For this review, take the finished solid that the model builds, in its own axes (mm). Round coordinates to 2 decimals unless told otherwise and drop trailing zeros. Write each loop counter-clockwise with the first axis right and the second up, starting at its lowest first coordinate (ties: lowest second). Pieces come first, ordered by that corner, then holes. Notation, with made-up numbers: M 18,8.5 L 53,8.5 A30 ccw 53,46.5 Z; hole C -37.5,50 d5. An arc over 180 degrees is marked long. Write each question's results on one line, items separated by ' | '. Start each with the question number.
```python
from build123d import *

# Parameters (mm, degrees)
BOSS_EXTRUDE1_DEPTH       = 1.5
FILLET1_R                 = 4
F_3_0MM_DOWEL_HOLE2_D     = 3
F_3_0MM_DOWEL_HOLE2_DEPTH = 17.29
F_3_0MM_DOWEL_HOLE2_TIP   = 0.901290929


with BuildPart() as part:
    # Sketch1 → Boss-Extrude1 (new body)
    with BuildSketch(Plane(origin=(0, 0, 0), x_dir=(0, 0, -1), z_dir=(1, 0, 0))):
        with BuildLine():
            Line((164.111754286, 40.215722327), (-6.393348286, 40.215722327))
            ThreePointArc((-6.393348286, 40.215722327), (12.614416769, 26.195971709), (19.859203, 3.715722327))
            ThreePointArc((19.859203, 3.715722327), (12.614416769, -18.764527055), (-6.393348286, -32.784277673))
            Line((-6.393348286, -32.784277673), (164.111754286, -32.784277673))
            ThreePointArc((164.111754286, -32.784277673), (137.859203, 3.715722327), (164.111754286, 40.215722327))
        make_face()
    extrude(amount=BOSS_EXTRUDE1_DEPTH)

    # Fillet1
    fillet1_edges = [part.edges().sort_by_distance(p)[0] for p in [
        (0.75, -32.784277673, -164.111754286),
        (0.75, -32.784277673, 6.393348286),
        (0.75, 40.215722327, 6.393348286),
        (0.75, 40.215722327, -164.111754286),
    ]]
    fillet(fillet1_edges, radius=FILLET1_R)

    # Ø3.0mm Dowel Hole2
    with Locations(Plane(origin=(1.5, 0, 0), x_dir=(0, 0, -1), z_dir=(1, 0, 0))):
        with Locations((8.745330875, 36.215722327), (148.973075124, 36.215722327), (148.973075124, -28.784277673), (8.745330875, -28.784277673), (43.745330875, 36.215722327), (113.973075124, -28.784277673)):
            Hole(F_3_0MM_DOWEL_HOLE2_D / 2, depth=F_3_0MM_DOWEL_HOLE2_DEPTH)
            with Locations((0, 0, -(F_3_0MM_DOWEL_HOLE2_DEPTH + F_3_0MM_DOWEL_HOLE2_TIP / 2))):  # 118° drill point
                Cone(0, F_3_0MM_DOWEL_HOLE2_D / 2, F_3_0MM_DOWEL_HOLE2_TIP, mode=Mode.SUBTRACT)


solid = part.part
```
Item 1: We need section C-C on y = 31. State the section outline as (x, z) points.
Item 2: Mouldability with a two-part tool opening along Z and no side actions: class faces 1 (the flat face through (0, 4, -78)), 2 (the cylindrical face through (0.74, -29.36, -112.59)), 3 (the cylindrical face through (0.74, 3.246, -137.862)) as pulls with the +Z half, pulls with the -Z half, needs draft (parallel to the pull), parting line crosses it, or undercut.
Item 3: We need section B-B on y = 0.5. State the section outline as (x, z) points, then the cut area to 3 significant figures.
Item 4: Insertion check: P1, Ø2.5, axis at y = 36.22, z = -43.75, coming from the +X side. The pin has a flat end and moves straight along its axis. Give the tip position at first contact, or say it passes through.
Item 5: We need section A-A on x = 1. State the section outline as (y, z) points.
Item 6: For probe 1 along Y at (x, z) = (1, -16); probe 2 along Y at (x, z) = (0.2, -142.5); probe 3 along Z at (x, y) = (0.7, -14), list the stretches that pass through material, from the lowest coordinate up.
Numbers:
1) outline: M 0,-149.2 L 1.5,-149.2 L 1.5,-8.52 L 0,-8.52 Z
2) face 1: needs draft | face 2: undercut | face 3: pulls with the -Z half
3) outline: M 0,-137.99 L 1.5,-137.99 L 1.5,-19.72 L 0,-19.72 Z | area: 177 mm^2
4) P1: passes through
5) outline: M -32.78,-148.97 A4 ccw -25.73,-151.55 A38.5 cw 33.16,-151.55 A4 ccw 40.22,-148.97 L 40.22,-8.75 A4 ccw 33.16,-6.17 A38.5 cw -25.73,-6.17 A4 ccw -32.78,-8.75 Z; hole C -28.78,-148.97 d3; hole C -28.78,-113.97 d3; hole C -28.78,-8.75 d3; hole C 36.22,-148.97 d3; hole C 36.22,-43.75 d3; hole C 36.22,-8.75 d3
6) probe 1: y = -32.78 to -13.09, 20.52 to 40.22 | probe 2: y = -32.78 to -14.61, 22.04 to 40.22 | probe 3: z = -142.18 to -15.54
